Could you check a few things on this model? Use its own coordinates, in mm. A direction names the side the tool comes from. Coordinates: 2 decimals unless noted, no trailing zeros. Loops run counter-clockwise (first coordinate to the right, second up) from the corner with the lowest first, then second, coordinate; pieces in that order, holes last. Notation, with made-up numbers: (50.25, 21.25) -> (81.25, 21.25) arc R20 cw to (81.25, 28.25) -> close; hole circle Ø1 at (-35.5, -31.5). An arc over 180 degrees is marked (long way). One line per question, with ' | ' between items.
Autodesk Inventor part; units mm, degrees
ref_plane "YZ Plane" through (0, 0, 0) normal (1, 0, 0) x (0, 1, 0)
ref_plane "XZ Plane" through (0, 0, 0) normal (0, 1, 0) x (-1, 0, 0)
ref_plane "XY Plane" through (0, 0, 0) normal (0, 0, 1) x (1, 0, 0)
sketch "Sketch1" plane through (0, 0, 0) normal (0, 0, 1) x (1, 0, 0)
  circle A0 centre (0, 0) radius 50
  dimension "d0" = 100
extrude "Extrusion1" add sketch "Sketch1" along normal blind 2000
sketch "Sketch2" plane through (0, 0, 0) normal (1, 0, 0) x (0, 1, 0)
  line L0 (50, 0) -> (-50, 0)
  arc A0 (-31.5648, -59.3002) -> (32.3259, -59.3002) centre (0.3805, -45) ccw
  line L1 (32.3259, -59.3002) -> (45.3805, 0)
  circle A1 centre (0.3805, -45) radius 17.5
  line L2 (-45, 0) -> (-31.5648, -59.3002)
  point P0 (0, 0)
  point P1 (0, 0)
  dimension "d3" = 35
  dimension "d4" = 35
  dimension "d5" = 45
  dimension "d6" = 45
  dimension "d7" = 45
extrude "Extrusion2" add sketch "Sketch2" along normal mid plane 30
shell "Shell1" thickness 30 removed faces 1 at (9.39, -8.8667, 2000)
properties part number "Parth_Cylinder2"
Q1. For pin 1 (3 mm diameter, centred on y = -10, z = 1777.5, fed in from -X); pin 2 (24 mm diameter, centred on y = 7.5, z = -51.5, fed in from +X); pin 3 (4 mm diameter, centred on y = 6, z = 297, fed in from +X); pin 4 (8 mm diameter, centred on y = 1, z = 1179, fed in from +X), each with a flat end and sliding along its axis, tell me the tip position at first contact or that it passes through.
Values follow:
pin 1: stops at x = -49.27 | pin 2: stops at x = 15 | pin 3: stops at x = 49.84 | pin 4: stops at x = 50
Q2. Imagine slicing it at C-C on z = 861. Write out the boundary of the cut face in (x, y), plus the area to 3 significant figures.
Values follow:
outline: circle Ø100 at (0, 0); hole circle Ø40 at (0, 0) | area: 6,600 mm2
Q3. Imagine slicing it at A-A on y = 0. Write out the boundary of the cut face in (x, z).
Values follow:
outline: (-50, 0) -> (-15, 0) -> (-15, -27.5) -> (15, -27.5) -> (15, 0) -> (50, 0) -> (50, 2000) -> (20, 2000) -> (20, 30) -> (-20, 30) -> (-20, 2000) -> (-50, 2000) -> close; (-15, -80) -> (15, -80) -> (15, -62.5) -> (-15, -62.5) -> close
Q4. Please list where these lines run through material, in increasing order: L1, parallel to Y at x = 0, z = 454; L2, parallel to X at y = -0.5, z = 1741.5; L3, parallel to Y at x = 4, z = 784.5. Write a range as [from, to].
Values follow:
L1: y = [-50, -20], [20, 50] | L2: x = [-50, -19.99], [19.99, 50] | L3: y = [-49.84, -19.6], [19.6, 49.84]
Q5. Imagine slicing it at B-B on x = 0. Write out the boundary of the cut face in (y, z), plus the area to 3 significant figures.
Values follow:
outline: (-50, 0) -> (-45, 0) -> (-31.56, -59.3) arc R35 ccw to (32.33, -59.3) -> (45.38, 0) -> (50, 0) -> (50, 2000) -> (20, 2000) -> (20, 30) -> (-20, 30) -> (-20, 2000) -> (-50, 2000) -> close; hole circle Ø35 at (0.38, -45) | area: 126,000 mm2
Q6. For faces 1 (the face through (-15, 0, -22)), 2 (the face through (-0.21, 9.788, -59.756)), which set-ups out of +Z, -Z, +X, -X, +Y, -Y let a thin tool reach every point of the face, with its end or its side?
Values follow:
face 1: -Z, -X, +Y, -Y | face 2: +X, -X
Q7. We'd pull the mould along Y, two halves only. Please class faces 3 (the face through (-4.336, 19.524, 1001.21)), 4 (the face through (15, 0, -22)), 5 (the face through (47.69, -15.02, 986)), 6 (the face through (0, 0, 30)): released by +Y, released by -Y, zero draft, split by the parting line, or undercut.
Values follow:
face 3: undercut | face 4: zero draft | face 5: split by the parting line | face 6: undercut
